```python
from build123d import *

# Parameters (mm, degrees)
SKETCH1_W           = 40
SKETCH1_H           = 52.3
SKETCH1_R           = 2.75
BOSS_EXTRUDE1_DEPTH = 12
SKETCH2_R           = 11
CUT_EXTRUDE1_DEPTH  = 8
SKETCH6_W           = 25
SKETCH6_H           = 40
BOSS_EXTRUDE3_DEPTH = 20
FILLET1_R           = 2
FILLET2_R           = 2
SKETCH7_R           = 4
CUT_EXTRUDE2_DEPTH  = 35


with BuildPart() as part:
    # Sketch1 → Boss-Extrude1 (new body)
    with BuildSketch(Plane.XY):
        Rectangle(SKETCH1_W, SKETCH1_H)
        with Locations((13, 16.9975)):
            Circle(SKETCH1_R, mode=Mode.SUBTRACT)
        with Locations((13, -16.9975)):
            Circle(SKETCH1_R, mode=Mode.SUBTRACT)
    extrude(amount=BOSS_EXTRUDE1_DEPTH)

    # Sketch2 → Cut-Extrude1 (cut)
    with BuildSketch(Plane.XY.offset(12)):
        Circle(SKETCH2_R)
    extrude(amount=-CUT_EXTRUDE1_DEPTH, mode=Mode.SUBTRACT)

    # Sketch6 → Boss-Extrude3 (add)
    with BuildSketch(Plane.ZY.offset(15)):
        with Locations((12.5, 0)):
            Rectangle(SKETCH6_W, SKETCH6_H)
    extrude(amount=BOSS_EXTRUDE3_DEPTH)

    # Fillet1
    fillet1_edges = [part.edges().sort_by_distance(p)[0] for p in [
        (-20, 20, 6),
        (-20, -20, 6),
    ]]
    fillet(fillet1_edges, radius=FILLET1_R)

    # Fillet2
    fillet2_edges = [part.edges().sort_by_distance(p)[0] for p in [
        (-15, 0, 12),
    ]]
    fillet(fillet2_edges, radius=FILLET2_R)

    # Sketch7 → Cut-Extrude2 (cut)
    with BuildSketch(Plane.XZ.offset(20)):
        with Locations((-25, 15)):
            Circle(SKETCH7_R)
    extrude(amount=-CUT_EXTRUDE2_DEPTH, mode=Mode.SUBTRACT)


solid = part.part
```
The model under review builds one solid part; all positions refer to its coordinate system, in mm. A direction names the side the tool comes from. Give positions to 0.01 mm unless a question says otherwise; leave off trailing zeros. Write each loop counter-clockwise with the first axis right and the second up, starting at its lowest first coordinate (ties: lowest second). Pieces come first, ordered by that corner, then holes.
(1) Consider section C-C, the plane x = 0. Give the boundary of the cut face in (y, z).
(2) Consider section B-B, the plane y = 0. Give the boundary of the cut face in (x, z), and give its area (3 significant figures).
(3) To check wall thickness, follow L1, parallel to Y at x = 13, z = 8; L2, parallel to Y at x = 0, z = 10; L3, parallel to Y at x = -31.5, z = 11. State the ranges of each line that lie inside material, in increasing order.
(4) Tool access review of faces 1 (the cylindrical face through (-27.95, -2.75, 17.7)), 2 (the flat face through (-20, -24, 6)), 3 (the flat face through (-20, 24, 6)), 4 (the flat face through (-15, 0, 19)): name each direction out of +Z, -Z, +X, -X, +Y, -Y from which nothing blocks a thin tool from reaching the whole face with its end or side.
(5) For P1, Ø3.5, axis at y = 25, z = 4.5, coming from the -X side; P2, Ø21, axis at x = 3.5, y = 8.5, coming from the +Z side; P3, Ø4, axis at x = -20.5, z = 15, coming from the -Y side, all flat-tipped, find the tip position at first contact; note any pin that passes through.
(6) Consider section D-D, the plane z = 7. Give the boundary of the cut face in (x, y), and give its area (3 significant figures).
(7) Consider section A-A, the plane x = 13. Give the boundary of the cut face in (y, z).
(8) The part is to be moulded in two halves that separate along X. For faces 5 (the flat face through (-29, -20, 12)), 6 (the flat face through (0, 0, 4)), 7 (the cylindrical face through (-20.6, -20.57, 5.92)), 8 (the cylindrical face through (-2.38, -10.74, 8.06)), say which applies: released by +X, released by -X, zero draft, split by the parting line, or undercut.
Returned:
1. outline: (-26.15, 0) - (26.15, 0) - (26.15, 12) - (11, 12) - (11, 4) - (-11, 4) - (-11, 12) - (-26.15, 12) - close
2. outline: (-35, 0) - (20, 0) - (20, 12) - (11, 12) - (11, 4) - (-11, 4) - (-11, 12) - (-13, 12) arc R2 cw to (-15, 14) - (-15, 25) - (-35, 25) - close; hole circle Ø8 at (-25, 15)
2. area: 695 mm2
3. L1: y = -26.15 to -19.75, -14.25 to 14.25, 19.75 to 26.15
3. L2: y = -26.15 to -11, 11 to 26.15
3. L3: y = -20 to 20
4. face 1: -Y
4. face 2: +Z, -Z, -X, -Y
4. face 3: +Z, -Z, -X, +Y
4. face 4: +Z, +X, +Y, -Y
5. P1: stops at x = -20
5. P2: stops at z = 12
5. P3: stops at y = -20
6. outline: (-35, -20) - (-22, -20) arc R2 cw to (-20, -22) - (-20, -26.15) - (20, -26.15) - (20, 26.15) - (-20, 26.15) - (-20, 22) arc R2 cw to (-22, 20) - (-35, 20) - close; hole circle Ø22 at (0, 0); hole circle Ø5.5 at (13, -17); hole circle Ø5.5 at (13, 17)
6. area: 2,270 mm2
7. outline: (-26.15, 0) - (-19.75, 0) - (-19.75, 12) - (-26.15, 12) - close; (-14.25, 0) - (14.25, 0) - (14.25, 12) - (-14.25, 12) - close; (19.75, 0) - (26.15, 0) - (26.15, 12) - (19.75, 12) - close
8. face 5: zero draft
8. face 6: undercut
8. face 7: released by -X
8. face 8: undercut
